Read the model definition and answer for the solid it produces. Units are mm, in the model's axes. A direction names the side the tool comes from. Give positions to 0.01 mm unless a question says otherwise; leave off trailing zeros. Loops run counter-clockwise (first coordinate to the right, second up) from the corner with the lowest first, then second, coordinate; pieces in that order, holes last. Notation, with made-up numbers: (-4.75, -24) - (51.25, -24) arc R19 cw to (51.25, 12) - close; hole circle Ø6 at (49, 37.5). An arc over 180 degrees is marked (long way). Use a Markdown table: item, result. Add a question column.
Item 1: A cutting plane is placed at B-B (y = 3.5). Determine the outline of the cut face in (x, z), plus the area to 4 significant figures.
Item 2: A cutting plane is placed at D-D (z = -26). Determine the outline of the cut face in (x, y).
Item 3: Each of these flat-tipped pins is pushed along its axis until it touches: P1, Ø1, axis at x = -15, z = 4, coming from the -Y side; P2, Ø2, axis at x = 13.5, z = -2.5, coming from the +Y side; P3, Ø1.2, axis at x = 13.5, y = 17, coming from the +Z side. Where does it stop, or does it pass through?
Item 4: A cutting plane is placed at A-A (z = -13). Determine the outline of the cut face in (x, y), plus the area to 3 significant figures.
Item 5: A cutting plane is placed at C-C (x = -6.5). Determine the outline of the cut face in (y, z), plus the area to 3 significant figures.
Item 6: Which of the six approach directions +Z, -Z, +X, -X, +Y, -Y give full straight-line access (tool end or side, diameter ignored) to faces 1 (the face through (-16.74, 19.39, -32.36)), 2 (the face through (-5, -12, -30)), 3 (the face through (0, -19, 22)), 4 (the face through (-14.726, 16.316, 24.612)), 5 (the face through (16.89, 19.24, -32.36))?
Item 7: Consider probe 1 along Z at (x, y) = (0, -20); probe 2 along X at (y, z) = (-14, -18); probe 3 along Y at (x, z) = (-4.5, -15). Determine where each line is inside the solid, lowest interval first. Write a range as [from, to].
Item 8: For a pull along X with two mould halves and no side action, classify faces 6 (the face through (13, -9, -16.5)), 7 (the face through (-9, -9, -32.5)), 8 (the face through (-20, -5, 0)) as +X half, -X half, draft (parallel to the pull), parting line (faces both ways), or undercut.
Autodesk Inventor part; units mm, degrees
ref_plane "YZ Plane" through (0, 0, 0) normal (1, 0, 0) x (0, 1, 0)
ref_plane "XZ Plane" through (0, 0, 0) normal (0, 1, 0) x (-1, 0, 0)
ref_plane "XY Plane" through (0, 0, 0) normal (0, 0, 1) x (1, 0, 0)
sketch "Skizze1" plane through (0, 0, 0) normal (0, 0, 1) x (1, 0, 0)
  circle A0 centre (0, 3.5) radius 14
  line L0 (-20, -22.5) -> (20, -22.5)
  line L1 (20, -22.5) -> (20, 12.5)
  line L2 (10, 22.5) -> (-10, 22.5)
  line L3 (-20, 12.5) -> (-20, -22.5)
  arc A1 (-10, 22.5) -> (-20, 12.5) centre (-10, 12.5) ccw
  arc A2 (20, 12.5) -> (10, 22.5) centre (10, 12.5) ccw
  dimension "d0" = 28
  dimension "d3" = 10
  dimension "d13" = 19
extrude "Extrusion1" add sketch "Skizze1" along normal mid plane 65
sketch "Skizze2" plane through (0, 0, 32.5) normal (0, 0, 1) x (1, 0, 0)
  circle A0 centre (0, 3.5) radius 18 construction
  circle A1 centre (0, -14.5) radius 2.5
  line L0 (-18, -14.5) -> (18, -14.5)
  line L1 (18, -14.5) -> (18, 21.5)
  line L2 (18, 21.5) -> (-18, 21.5)
  line L3 (-18, 21.5) -> (-18, -14.5)
  line L4 (-18, -14.5) -> (18, 21.5) construction
  line L5 (18, -14.5) -> (-18, 21.5) construction
  circle A2 centre (12.7279, 16.2279) radius 2
  circle A3 centre (12.7279, -9.2279) radius 2
  circle A4 centre (-12.7279, -9.2279) radius 2
  circle A5 centre (-12.7279, 16.2279) radius 2
  circle A6 centre (0, 3.5) radius 14
  dimension "d6" = 36
  dimension "d7" = 5
  dimension "d8" = 4
  dimension "d9" = 4
  dimension "d10" = 4
  dimension "d11" = 4
extrude "Extrusion2" cut sketch "Skizze2" against normal blind 16 contours L0 A1 | A1 L0 | A2 | A3 | A4 | A5
sketch "Skizze3" plane through (0, 0, 32.5) normal (0, 0, 1) x (1, 0, 0)
  line L0 (-3, -17) -> (3, -17)
  line L1 (5, -15) -> (5, -12)
  line L2 (5, -12) -> (-5, -12)
  line L3 (-5, -12) -> (-5, -15)
  circle A0 centre (0, -14.5) radius 2.5
  line L4 (-5, -17) -> (5, -12) construction
  line L5 (5, -17) -> (-5, -12) construction
  circle A1 centre (0, 3.5) radius 14
  line L6 (-5, -12) -> (5, -12)
  line L7 (5, -12) -> (5, -9.5767)
  line L8 (5, -9.5767) -> (-5, -9.5767)
  line L9 (-5, -9.5767) -> (-5, -12)
  arc A2 (-5, -15) -> (-3, -17) centre (-3, -15) ccw
  arc A3 (3, -17) -> (5, -15) centre (3, -15) ccw
  point P0 (0, 0)
  dimension "d16" = 10
  dimension "d17" = 2
extrude "Extrusion3" cut sketch "Skizze3" against normal blind 5 contours A2 L3 L2 A0 L0 | A0 L2 L1 A3 L0 | A0 | L2 L9 A1 L7
sketch "Skizze4" plane through (-20, -22.5, 32.5) normal (0, -1, 0) x (1, 0, 0)
  line L0 (17.5, -16) -> (22.5, -16)
  line L1 (17.5, -5) -> (17.5, -16)
  line L2 (22.5, -5) -> (22.5, -16)
  line L3 (17.5, -16) -> (22.5, -16)
  line L4 (22.5, -16) -> (22.5, -10.5)
  line L5 (22.5, -10.5) -> (17.5, -10.5)
  line L6 (17.5, -10.5) -> (17.5, -16)
  line L7 (20, -16) -> (20, -10.5) construction
  line L8 (21.75, -14.25) -> (21.75, -12.25)
  line L9 (18.25, -12.25) -> (18.25, -14.25)
  arc A0 (18.25, -14.25) -> (21.75, -14.25) centre (20, -14.25) ccw
  arc A1 (21.75, -12.25) -> (18.25, -12.25) centre (20, -12.25) ccw
  point P0 (20, -32.5)
  point P1 (20, -13.25)
  dimension "d20" = 5.5
  dimension "d21" = 3.5
extrude "Extrusion4" cut sketch "Skizze4" against normal up to surface contours A0 L9 A1 L8
sketch "Skizze5" plane through (-20, -22.5, 32.5) normal (0, -1, 0) x (1, 0, 0)
  line L0 (40, 0) -> (40, -65)
  line L1 (0, -22.5) -> (40, -22.5)
  line L2 (40, -22.5) -> (40, -42.5)
  line L3 (40, -42.5) -> (0, -42.5)
  line L4 (0, -42.5) -> (0, -22.5)
  line L5 (0, -22.5) -> (40, -42.5) construction
  line L6 (40, -22.5) -> (0, -42.5) construction
  point P0 (20, -32.5)
  dimension "d24" = 20
extrude "Extrusion5" cut sketch "Skizze5" against normal blind 1
sketch "Skizze6" plane through (-20, -21.5, 32.5) normal (0, -1, 0) x (1, 0, 0)
  point P0 (20, -32.5)
hole "Bohrung1" at (0, -21.5, 0) direction (0, 1, 0) diameter 4.917 depth 9
ref_plane "Arbeitsebene1" through (0, 0, 0) normal (0, 0, 1) x (1, 0, 0)
mirror "Spiegeln1" about plane through (0, 0, 0) normal (0, 0, 1) of "Extrusion3", "Extrusion2", "Extrusion4"
chamfer "Fasen1" distance 0.5 angle 45 22 edges at (20, -5, 32.5) (17.0711, 19.5711, 32.5) (0, 22.5, 32.5) (-17.0711, 19.5711, 32.5) (-20, -5, 32.5) (20, -22.5, 21.25) (20, -21.5, 0) (20, -22.5, -21.25) (0, -22.5, 32.5) (-20, -22.5, 21.25) (-20, -22.5, -21.25) (17.0711, 19.5711, -32.5) (20, -5, -32.5) (0, 22.5, -32.5) (-17.0711, 19.5711, -32.5) (-20, -5, -32.5) (-20, -21.5, 0) (-20, -22, 10) (-20, -22, -10) (20, -22, -10) (20, -22, 10) (0, -22.5, -32.5)
properties part number "sf_Cylinder_1"
Geometry says:
| question | item | result |
|---|---|---|
| 1 | outline | (-20, -32) - (-19.5, -32.5) - (-14, -32.5) - (-14, 32.5) - (-19.5, 32.5) - (-20, 32) - close; (14, -32.5) - (19.5, -32.5) - (20, -32) - (20, 32) - (19.5, 32.5) - (14, 32.5) - close |
| 1 | area | 779.5 mm² |
| 2 | outline | (-20, -22) - (-19.5, -22.5) - (19.5, -22.5) - (20, -22) - (20, 12.5) arc R10 ccw to (10, 22.5) - (-10, 22.5) arc R10 ccw to (-20, 12.5) - close; hole circle Ø4 at (-12.73, -9.23); hole circle Ø4 at (-12.73, 16.23); hole circle Ø28 at (0, 3.5); hole circle Ø5 at (0, -14.5); hole circle Ø4 at (12.73, -9.23); hole circle Ø4 at (12.73, 16.23) |
| 3 | P1 | y = -21.5 |
| 3 | P2 | y = 22.18 |
| 3 | P3 | z = 16.5 |
| 4 | outline | (-20, -22) - (-19.5, -22.5) - (19.5, -22.5) - (20, -22) - (20, 12.5) arc R10 ccw to (10, 22.5) - (-10, 22.5) arc R10 ccw to (-20, 12.5) - close; hole circle Ø28 at (0, 3.5) |
| 4 | area | 1,140 mm² |
| 5 | outline | (-22.5, -32) - (-22, -32.5) - (-8.9, -32.5) - (-8.9, 32.5) - (-22, 32.5) - (-22.5, 32) - (-22.5, 10) - (-21.5, 10) - (-21.5, -10) - (-22.5, -10) - close; (15.9, -32.5) - (22, -32.5) - (22.5, -32) - (22.5, 32) - (22, 32.5) - (15.9, 32.5) - close |
| 5 | area | 1,290 mm² |
| 6 | face 1 | -Z, -X, +Y |
| 6 | face 2 | -Z |
| 6 | face 3 | -Y |
| 6 | face 4 | +Z |
| 6 | face 5 | -Z, +X, +Y |
| 7 | probe 1 | [-32.5, -22], [-16.5, -2.46], [2.46, 16.5], [22, 32.5] |
| 7 | probe 2 | [-20, -2.45], [2.45, 20] |
| 7 | probe 3 | [-22.5, -9.76], [16.76, 22.5] |
| 8 | face 6 | undercut |
| 8 | face 7 | draft |
| 8 | face 8 | -X half |
